Answer from the drawing. Dimensions are ordinates in mm from the lowest x, y and z of the part. A direction names the side the tool comes from. Round coordinates to 2 decimals unless told otherwise and drop trailing zeros. Write each loop counter-clockwise with the first axis right and the second up, starting at its lowest first coordinate (ties: lowest second). Pieces come first, ordered by that corner, then holes. Notation, with made-up numbers: (39, 85.5) - (72, 85.5) arc R19 ccw to (72, 118.5) - close; hole circle Ø4 at (17, 6.25). An arc over 180 degrees is marked (long way). Answer as a JSON object with one key per item and string values.
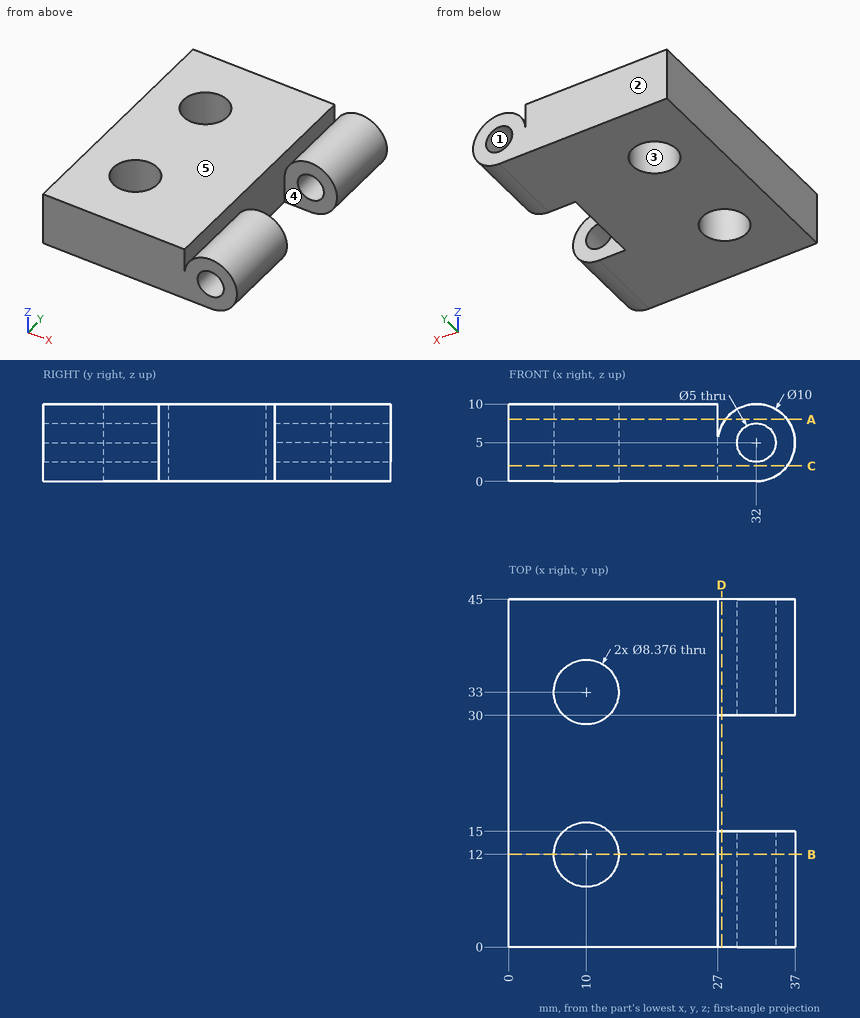
Item 1: A cutting plane is placed at B-B (y = 12). Write down the section's boundary in (x, z), and give its area (3 significant figures).
Results found:
{"outline": "(0, 0) - (5.81, 0) - (5.81, 10) - (0, 10) - close; (14.19, 0) - (32, 0) arc R5 ccw (long way) to (27, 5) - (27, 10) - (14.19, 10) - close; hole circle Ø5 at (32, 5)", "area": "251 mm²"}
Item 2: A cutting plane is placed at D-D (x = 27.5). Write down the section's boundary in (y, z), and give its area (3 significant figures).
Results found:
{"outline": "(0, 0) - (15, 0) - (15, 7.18) - (0, 7.18) - close; (30, 0) - (45, 0) - (45, 7.18) - (30, 7.18) - close", "area": "215 mm²"}
Item 3: Each of these flat-tipped pins is pushed along its axis until it touches: P1, Ø2, axis at y = 37.5, z = 2.5, coming from the +X side; P2, Ø3, axis at x = 33.5, z = 3.5, coming from the +Y side; P3, Ø3, axis at y = 20, z = 1.5, coming from the +X side; P4, Ø6, axis at y = 8, z = 1.5, coming from the +X side. Where does it stop, or does it pass through?
Results found:
{"P1": "x = 36.77", "P2": "y = 45", "P3": "x = 27", "P4": "x = 36.97"}
Item 4: A cutting plane is placed at C-C (z = 2). Write down the section's boundary in (x, y), and give its area (3 significant figures).
Results found:
{"outline": "(0, 0) - (36, 0) - (36, 15) - (27, 15) - (27, 30) - (36, 30) - (36, 45) - (0, 45) - close; hole circle Ø8.38 at (10, 12); hole circle Ø8.38 at (10, 33)", "area": "1,370 mm²"}
Item 5: Consider line 1 along Y through (x, z) = (10, 4.5); line 2 along Y through (x, z) = (29.5, 3.5); line 3 along X through (y, z) = (34, 6.5). Determine where each line is inside the solid, lowest interval first.
Results found:
{"line 1": "0 to 7.81, 16.19 to 28.81, 37.19 to 45", "line 2": "0 to 15, 30 to 45", "line 3": "0 to 5.93, 14.07 to 27, 27.23 to 30, 34 to 36.77"}
Item 6: A cutting plane is placed at A-A (z = 8). Write down the section's boundary in (x, y), and give its area (3 significant figures).
Results found:
{"outline": "(0, 0) - (27, 0) - (27, 45) - (0, 45) - close; (28, 0) - (36, 0) - (36, 15) - (28, 15) - close; (28, 30) - (36, 30) - (36, 45) - (28, 45) - close; hole circle Ø8.38 at (10, 12); hole circle Ø8.38 at (10, 33)", "area": "1,340 mm²"}
Item 7: For the marked faces 4 and 5, determine the directions among +Z, -Z, +X, -X, +Y, -Y from which every point of the face is accessible in a straight line to the end or side of a thin tool.
Results found:
{"face 4": "+Z, -Z, +X", "face 5": "+Z, +X, -X, +Y, -Y"}
Item 8: Determine the mould class of the marked faces 1, 2 and 3 for opening direction Y: pulls with the +Y half, pulls with the -Y half, needs draft (parallel to the pull), parting line crosses it, or undercut.
Results found:
{"face 1": "needs draft", "face 2": "pulls with the +Y half", "face 3": "undercut"}
